Check sheet for the modelled part. Datum: model origin and axes. Units: mm. Face numbers are marked on the shaded views. A direction names the side the tool comes from. Coordinates: 2 decimals unless noted, no trailing zeros. Loops run counter-clockwise (first coordinate to the right, second up) from the corner with the lowest first, then second, coordinate; pieces in that order, holes last. Notation, with made-up numbers: (52, 15) -> (97, 15) arc R26 ccw to (97, 49) -> close; hole circle Ø10 at (-30.75, 33). An arc over 180 degrees is marked (long way). Use CSV: the item, a comma, the result in double quotes. Start each with the question number.
1. Release check for a two-part mould opening along Y. For the marked faces 1, 2 and 3 record: pulls with the +Y half, pulls with the -Y half, needs draft (parallel to the pull), parting line crosses it, or undercut.
2. Sectioned sample at C-C, the plane z = -7. Record the cut outline in (x, y), and give its area (3 significant figures).
3. Gauge pin test, flat ends, axial feed: pin 1 (2.5 mm diameter, centred on y = 13, z = -23, fed in from -X); pin 2 (10 mm diameter, centred on x = -11.5, z = -4.5, fed in from -Y); pin 3 (5.5 mm diameter, centred on y = 7, z = -22, fed in from +X). Record the tip position at first contact, or that the pin passes through.
4. Set-up check for the marked faces 4, 5, 6, 7 and 8: record each of +Z, -Z, +X, -X, +Y, -Y from which the full face is reachable in a straight line by a thin tool's end or side.
5. Sectioned sample at B-B, the plane x = 0. Record the cut outline in (y, z), and give its area (3 significant figures).
6. Sectioned sample at D-D, the plane x = 25. Record the cut outline in (y, z), and give its area (3 significant figures).
7. Sectioned sample at A-A, the plane y = 45.5. Record the cut outline in (x, z).
8. Thickness scan on L1, parallel to Y at x = -25, z = -28; L2, parallel to X at y = 39, z = -3; L3, parallel to Y at x = -7, z = -4.5. Record the ranges inside material, lowest first.
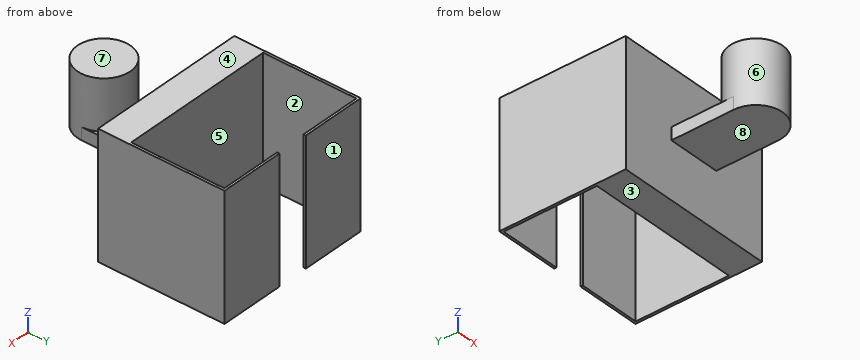
```python
from build123d import *

# Parameters (mm, degrees)
SKETCH1_R           = 10.777569686
BOSS_EXTRUDE1_DEPTH = 25.4
SKETCH2_W           = 21.555139372
SKETCH2_H           = 25.4
BOSS_EXTRUDE2_DEPTH = 5.08
SKETCH6_W           = 65.44191557
SKETCH6_H           = 50.8
BOSS_EXTRUDE3_DEPTH = 51.639420176
SKETCH7_W           = 63.40856
SKETCH7_H           = 38.0746
CUT_EXTRUDE1_DEPTH  = 98.910026756
SKETCH8_W           = 12.6492
SKETCH8_H           = 0.915620176
CUT_EXTRUDE2_DEPTH  = 98.910026756


with BuildPart() as part:
    # Sketch1 → Boss-Extrude1 (new body)
    with BuildSketch(Plane.XY):
        Circle(SKETCH1_R)
    extrude(amount=-BOSS_EXTRUDE1_DEPTH)

    # Sketch2 → Boss-Extrude2 (add)
    with BuildSketch(Plane(origin=(0, 0, -25.4), x_dir=(-1, 0, 0), z_dir=(0, 0, -1))):
        with Locations((0, 12.7)):
            Rectangle(SKETCH2_W, SKETCH2_H)
    extrude(amount=-BOSS_EXTRUDE2_DEPTH)

    # Sketch6 → Boss-Extrude3 (add)
    with BuildSketch(Plane(origin=(0, 25.4, 0), x_dir=(1, 0, 0), z_dir=(0, 1, 0))):
        with Locations((0, 22.86)):
            Rectangle(SKETCH6_W, SKETCH6_H)
    extrude(amount=BOSS_EXTRUDE3_DEPTH)

    # Sketch7 → Cut-Extrude1 (cut, through all)
    with BuildSketch(Plane.XY.offset(2.54)):
        with Locations((0, 57.0865)):
            Rectangle(SKETCH7_W, SKETCH7_H)
    extrude(amount=-CUT_EXTRUDE1_DEPTH, mode=Mode.SUBTRACT)

    # Sketch8 → Cut-Extrude2 (cut, through all)
    with BuildSketch(Plane.XY.offset(2.54)):
        with Locations((0, 76.581610088)):
            Rectangle(SKETCH8_W, SKETCH8_H)
    extrude(amount=-CUT_EXTRUDE2_DEPTH, mode=Mode.SUBTRACT)


solid = part.part
```
Completed:
1,face 1,"pulls with the +Y half"
1,face 2,"undercut"
1,face 3,"needs draft"
2,outline,"(-32.72, 25.4) -> (32.72, 25.4) -> (32.72, 77.04) -> (6.32, 77.04) -> (6.32, 76.12) -> (31.7, 76.12) -> (31.7, 38.05) -> (-31.7, 38.05) -> (-31.7, 76.12) -> (-6.32, 76.12) -> (-6.32, 77.04) -> (-32.72, 77.04) -> close; circle Ø21.56 at (0, 0)"
2,area,"1,320 mm²"
3,pin 1,"x = -10.78"
3,pin 2,"y = -8.6"
3,pin 3,"x = 10.78"
4,face 4,"+Z, +X, -X, +Y, -Y"
4,face 5,"+Z, -Z"
4,face 6,"+Z"
4,face 7,"+Z, +X, -X, -Y"
4,face 8,"-Z, +X, -X, -Y"
5,outline,"(-10.78, -25.4) -> (25.4, -25.4) -> (25.4, -48.26) -> (38.05, -48.26) -> (38.05, 2.54) -> (25.4, 2.54) -> (25.4, -20.32) -> (10.78, -20.32) -> (10.78, 0) -> (-10.78, 0) -> close"
5,area,"1,260 mm²"
6,outline,"(25.4, -48.26) -> (38.05, -48.26) -> (38.05, 2.54) -> (25.4, 2.54) -> close; (76.12, -48.26) -> (77.04, -48.26) -> (77.04, 2.54) -> (76.12, 2.54) -> close"
6,area,"689 mm²"
7,outline,"(-32.72, -48.26) -> (-31.7, -48.26) -> (-31.7, 2.54) -> (-32.72, 2.54) -> close; (31.7, -48.26) -> (32.72, -48.26) -> (32.72, 2.54) -> (31.7, 2.54) -> close"
8,L1,"25.4 to 38.05, 76.12 to 77.04"
8,L2,"-32.72 to -31.7, 31.7 to 32.72"
8,L3,"-8.19 to 8.19, 25.4 to 38.05, 76.12 to 77.04"
